Verification items for the finished model (mm, model axes). A direction names the side the tool comes from. Coordinates: 2 decimals unless noted, no trailing zeros. Write each loop counter-clockwise with the first axis right and the second up, starting at its lowest first coordinate (ties: lowest second). Pieces come first, ordered by that corner, then holes. Notation, with made-up numbers: (30, 31) -> (86, 31) arc R28 ccw to (86, 51) -> close; hole circle Ø5 at (-32.5, 25). An arc over 180 degrees is marked (long way). Write item = value, one per line. Start each with the question number.
(1) Mould release check, pull along X, two halves, no side actions. Record for faces 4 (the face through (-17, -18, 1)), 5 (the face through (3.5, -23, 1)), 6 (the face through (31.359, -19.297, 1.014)), 7 (the face through (0, 29, 1)): released by +X, released by -X, zero draft, split by the parting line, or undercut.
(2) Gauge pin test, flat ends, axial feed: pin 1 Ø1.2 at (x, y) = (-12.5, 21.65) entering from +Z; pin 2 Ø0.6 at (x, z) = (0.5, 1) entering from -Y; pin 3 Ø0.6 at (x, z) = (25.5, 0.5) entering from -Y. Record the tip position at first contact, or that the pin passes through.
(3) Set-up check for faces 1 (the face through (-24, -20.5, 1)), 2 (the face through (24, 20.5, 1)), 3 (the face through (-3.5, -23, 1)): record each of +Z, -Z, +X, -X, +Y, -Y from which the full face is reachable in a straight line by a thin tool's end or side.
(4) Section check D-D (x = -9.5). Record the cut outline in (y, z).
(5) Section check A-A (y = 0). Record the cut outline in (x, z), plus the area to 3 significant figures.
(6) Material ranges on probe 1 along Y at (x, z) = (-12.5, 1.55); probe 2 along X at (y, z) = (-18.5, 0.2); probe 3 along X at (y, z) = (9.5, 0.3), recorded low to high. Write a range as [from, to].
(7) Section check C-C (y = -6). Record the cut outline in (x, z).
(8) Section check B-B (x = 19). Record the cut outline in (y, z), plus the area to 3 significant figures.
```python
from build123d import *

# Parameters (mm, degrees)
SKETCH1_R             = 18
BOSS_EXTRUDE1_DEPTH   = 2
SKETCH2_R             = 1.6
CUT_EXTRUDE1_DEPTH    = 2
F_2_0MM_DOWEL_HOLE1_D = 2
FILLET1_R             = 4
SKETCH_1_W            = 7
SKETCH_1_H            = 5
CUT_EXTRUDE_1_DEPTH   = 44.603325561
F_2_0MM_1_D           = 2


with BuildPart() as part:
    # Sketch1 → Boss-Extrude1 (new body)
    with BuildSketch(Plane.XY):
        with BuildLine():
            Line((-32.5, 20.5), (-20.512191497, 20.5))
            ThreePointArc((-20.512191497, 20.5), (0, 29), (20.512191497, 20.5))
            Line((20.512191497, 20.5), (32.5, 20.5))
            Line((32.5, 20.5), (32.5, -20.5))
            Line((32.5, -20.5), (20.512191497, -20.5))
            ThreePointArc((20.512191497, -20.5), (0, -29), (-20.512191497, -20.5))
            Line((-20.512191497, -20.5), (-32.5, -20.5))
            Line((-32.5, -20.5), (-32.5, 20.5))
        make_face()
        Circle(SKETCH1_R, mode=Mode.SUBTRACT)
    extrude(amount=BOSS_EXTRUDE1_DEPTH)

    # Sketch2 → Cut-Extrude1 (cut)
    with BuildSketch(Plane.XY.offset(2)):
        with Locations((-29, 14)):
            Circle(SKETCH2_R)
        with Locations((-29, -18)):
            Circle(SKETCH2_R)
        with Locations((29, -18)):
            Circle(SKETCH2_R)
        with Locations((29, 14)):
            Circle(SKETCH2_R)
    extrude(amount=-CUT_EXTRUDE1_DEPTH, mode=Mode.SUBTRACT)

    # Ø2.0mm Dowel Hole1 (through all)
    with Locations(Plane(origin=(-19, 19, 2), x_dir=(1, 0, 0), z_dir=(0, 0, 1))):
        with Locations((0, 0), (2, -2), (36, -2), (38, 0), (36, -36), (38, -38), (0, -38), (2, -36)):
            Hole(F_2_0MM_DOWEL_HOLE1_D / 2)

    # Fillet1
    fillet1_edges = [part.edges().sort_by_distance(p)[0] for p in [
        (-32.5, -20.5, 1),
        (-32.5, 20.5, 1),
        (32.5, 20.5, 1),
        (32.5, -20.5, 1),
    ]]
    fillet(fillet1_edges, radius=FILLET1_R)

    # 스케치1 → 컷-돌출1 (cut, through all)
    with BuildSketch(Plane(origin=(0, 0, 0), x_dir=(-1, 0, 0), z_dir=(0, 0, -1))):
        with Locations((0, -23)):
            Rectangle(SKETCH_1_W, SKETCH_1_H)
    extrude(amount=-CUT_EXTRUDE_1_DEPTH, mode=Mode.SUBTRACT)

    # Ø2.0mm 맞춤핀 구멍1 (through all)
    with Locations(Plane(origin=(12.5, 21.650635095, 0), x_dir=(-1, 0, 0), z_dir=(0, 0, -1))):
        with Locations((0, 0), (25, 0), (37.5, -21.650635095), (25, -43.30127019), (0, -43.30127019), (-12.5, -21.650635095)):
            Hole(F_2_0MM_1_D / 2)


solid = part.part
```
Response:
q1.face_4 = undercut
q1.face_5 = undercut
q1.face_6 = released by +X
q1.face_7 = split by the parting line
q2.pin_1 = through
q2.pin_2 = -29
q2.pin_3 = -20.5
q3.face_1 = +Z, -Z, -X, -Y
q3.face_2 = +Z, -Z, +X, +Y
q3.face_3 = +Z, -Z
q4.outline = (-27.4, 0) -> (-15.29, 0) -> (-15.29, 2) -> (-27.4, 2) -> close; (15.29, 0) -> (27.4, 0) -> (27.4, 2) -> (15.29, 2) -> close
q5.outline = (-32.5, 0) -> (-26, 0) -> (-26, 2) -> (-32.5, 2) -> close; (-24, 0) -> (-18, 0) -> (-18, 2) -> (-24, 2) -> close; (18, 0) -> (24, 0) -> (24, 2) -> (18, 2) -> close; (26, 0) -> (32.5, 0) -> (32.5, 2) -> (26, 2) -> close
q5.area = 50.0 mm2
q6.probe_1 = [-26.17, -22.65], [-20.65, -12.95], [12.95, 20.65], [22.65, 26.17]
q6.probe_2 = [-31.96, -30.52], [-27.48, -19.87], [-18.13, 18.13], [19.87, 27.48], [30.52, 31.96]
q6.probe_3 = [-32.5, -15.29], [15.29, 32.5]
q7.outline = (-32.5, 0) -> (-16.97, 0) -> (-16.97, 2) -> (-32.5, 2) -> close; (16.97, 0) -> (32.5, 0) -> (32.5, 2) -> (16.97, 2) -> close
q8.outline = (-21.91, 0) -> (-20, 0) -> (-20, 2) -> (-21.91, 2) -> close; (-18, 0) -> (18, 0) -> (18, 2) -> (-18, 2) -> close; (20, 0) -> (21.91, 0) -> (21.91, 2) -> (20, 2) -> close
q8.area = 79.6 mm2
